The listing builds one solid part. Answer for the finished solid, in the listing's coordinates (mm). Face numbers are marked on the shaded views. Coordinates: 2 decimals unless noted, no trailing zeros. Loops run counter-clockwise (first coordinate to the right, second up) from the corner with the lowest first, then second, coordinate; pieces in that order, holes last. Notation, with made-up numbers: (42, 1) - (65, 1) arc R27 ccw to (65, 31) - close; hole circle Ø1 at (-2, -10.5). An arc over 180 degrees is marked (long way). Put each result on its own line as item: value.
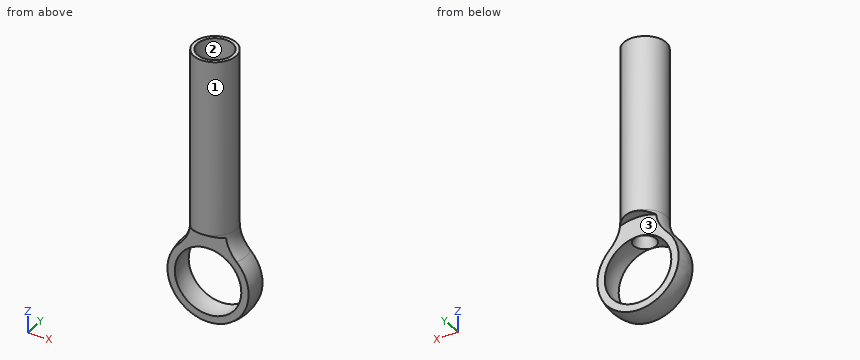
```python
from build123d import *

# Parameters (mm, degrees)
SHELL1_T           = -1.27
SKETCH2_R          = 1.5875
CUT_EXTRUDE2_DEPTH = 6.35
SKETCH3_R          = 4.7625
CUT_EXTRUDE3_DEPTH = 3.81


with BuildPart() as part:
    # Sketch1 → Revolve1 (revolve)
    with BuildSketch(Plane(origin=(0, 0, 0), x_dir=(1, 0, 0), z_dir=(0, 1, 0))):
        with BuildLine():
            Line((-1.905, -4.794144866), (-1.905, -20.542144866))
            Line((-1.905, -20.542144866), (0, -20.542144866))
            Line((0, -20.542144866), (0, 3.81))
            ThreePointArc((0, 3.81), (-3.498514306, 1.508806698), (-2.770909091, -2.614988109))
            ThreePointArc((-2.770909091, -2.614988109), (-2.129407802, -3.621698415), (-1.905, -4.794144866))
        make_face()
    revolve(axis=Axis((0, 0, -3.81), (0, 0, 1)))

    # Shell1
    shell1_openings = [part.faces().sort_by_distance(p)[0] for p in [
        (0, 0, 20.542144866),
    ]]
    offset(amount=SHELL1_T, openings=shell1_openings, kind=Kind.INTERSECTION)

    # Sketch4 → Cut-Revolve1 (revolve, cut)
    with BuildSketch(Plane(origin=(0, 0, 0), x_dir=(0, 0, -1), z_dir=(1, 0, 0))):
        with BuildLine():
            Line((0, 3.175), (0, -3.175))
            ThreePointArc((0, -3.175), (3.175, 0), (0, 3.175))
        make_face()
    revolve(axis=Axis((0, 3.175, 0), (0, -1, 0)), mode=Mode.SUBTRACT)

    # Sketch2 → Cut-Extrude2 (cut)
    with BuildSketch(Plane.XY.offset(20.542144866)):
        Circle(SKETCH2_R)
    extrude(amount=-CUT_EXTRUDE2_DEPTH, mode=Mode.SUBTRACT)

    # Sketch3 → Cut-Extrude3 (cut)
    with BuildSketch(Plane(origin=(0, 1.016, 0), x_dir=(1, 0, 0), z_dir=(0, 1, 0))):
        Circle(SKETCH3_R)
    cut_extrude3 = extrude(amount=CUT_EXTRUDE3_DEPTH, mode=Mode.SUBTRACT)

    # Mirror1: Cut-Extrude3 across plane
    add(cut_extrude3.mirror(Plane.ZX), mode=Mode.SUBTRACT)


solid = part.part
```
1) Straight lines are drawn through the part: L1, parallel to Y at x = 0, z = 17.5 (1 decimal); L2, parallel to Y at x = 0, z = 10.75 (3 decimals). For each, find the intervals that lie inside material, in ascending order. Write a range as [from, to].
Found:
L1: y = [-1.9, -1.6], [1.6, 1.9]
L2: y = [-1.905, -0.635], [0.635, 1.905]
2) The part is cut by section A-A (x = 0). State how many separate pieces and enclosed holes the cut face has, and give its area (3 significant figures).
Found:
separate pieces: 3
enclosed holes: 0
area: 30.2 mm^2
3) For a pull along Y with two mould halves and no side action, classify the marked faces 1, 2 and 3 as pulls with the +Y half, pulls with the -Y half, needs draft (parallel to the pull), parting line crosses it, or undercut.
Found:
face 1: parting line crosses it
face 2: undercut
face 3: pulls with the +Y half
4) The part is cut by section C-C (z = 3.5). Give the vertices of the cut face in (x, y).
Found:
outline: (-1.93, -1.02) - (1.93, -1.02) arc R2.18 ccw to (1.93, 1.02) - (-1.93, 1.02) arc R2.18 ccw to start; hole circle Ø1.66 at (0, 0)
5) Each of these flat-tipped pins is pushed along its axis until it touches: pin 1 (2 mm diameter, centred on x = 2, z = 6.5, fed in from -Y); pin 2 (3.5 mm diameter, centred on x = 1.5, z = -1, fed in from +Y); pin 3 (3.5 mm diameter, centred on x = -0.5, z = 2, fed in from -Y); pin 4 (3 mm diameter, centred on x = -0.5, z = 5.5, fed in from -Y). Where does it stop, or does it pass through?
Found:
pin 1: stops at y = -1.62
pin 2: stops at y = 1.02
pin 3: stops at y = -1.02
pin 4: stops at y = -1.91
